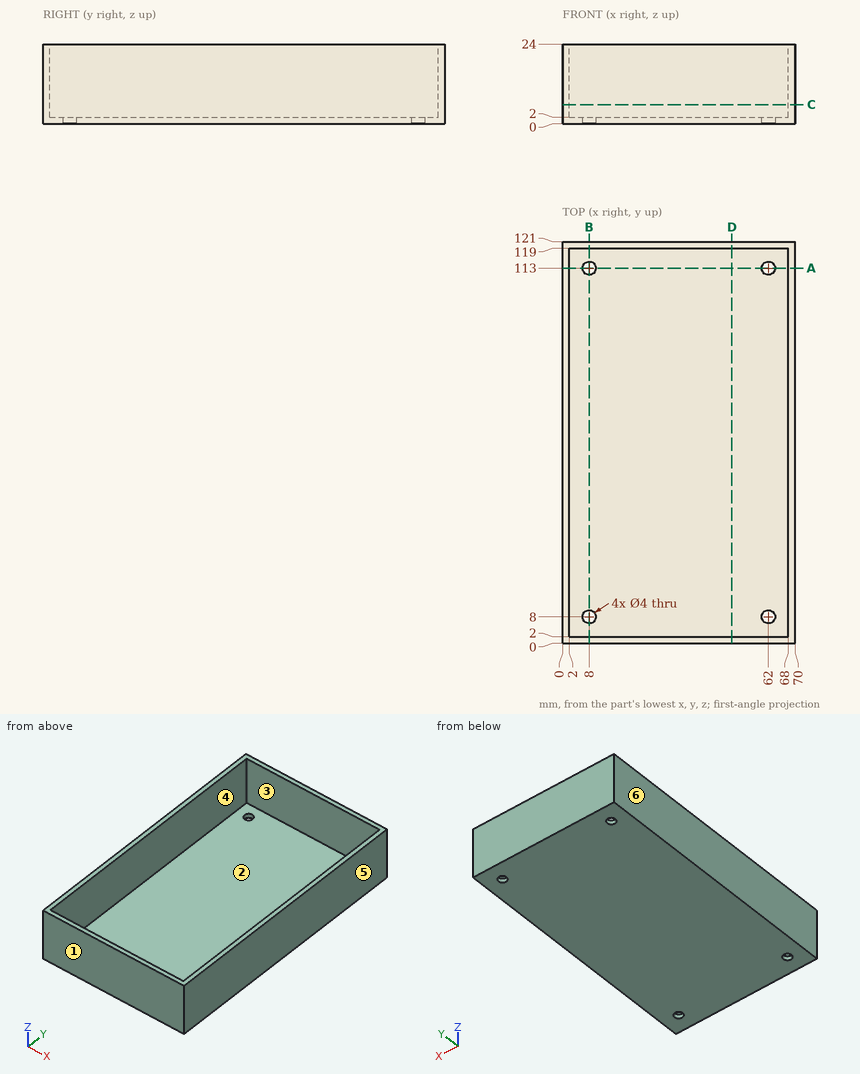
Part print with two shaded views. Sizes in mm from the minimum x, y, z corner. A direction names the side the tool comes from. Give positions to 0.01 mm unless a question says otherwise; leave off trailing zeros. Order: outer loops, then holes, each group sorted by start corner. A loop starts at its lowest first (then second) coordinate and runs counter-clockwise, first axis right, second up.
(1) Flat gauge pins, fed straight in: pin 1 (2.5 mm diameter, centred on x = 8, y = 8, fed in from -Z); pin 2 (8 mm diameter, centred on x = 49, y = 41.5, fed in from +Z). Where does each tip first touch, or does it go through?
(2) Saw through at A-A, the plane y = 113. Give the cut face in (x, z).
(3) Saw through at B-B, the plane x = 8. Give the cut face in (y, z), then the cut area to 3 significant figures.
(4) Drill centre lines: L1, parallel to Y at x = 62, z = 1.5; L2, parallel to Y at x = 7, z = 12; L3, parallel to X at y = 41.5, z = 6. Where is each one in solid material? Low to high.
(5) Saw through at C-C, the plane z = 5.75. Give the cut face in (x, y), then the cut area to 3 significant figures.
(6) Tool access for the marked faces 1 and 2: list every direction of +Z, -Z, +X, -X, +Y, -Y with a clear straight run to the whole face (end or side of a thin tool).
(7) Saw through at D-D, the plane x = 51. Give the cut face in (y, z).
(8) Mould opens along X. For the marked faces 3, 4, 5 and 6 say: released by +X, released by -X, zero draft, split by the parting line, or undercut.
Results found:
1. pin 1: passes through
1. pin 2: stops at z = 2
2. outline: (0, 0) - (6, 0) - (6, 2) - (2, 2) - (2, 24) - (0, 24) - close; (10, 0) - (60, 0) - (60, 2) - (10, 2) - close; (64, 0) - (70, 0) - (70, 24) - (68, 24) - (68, 2) - (64, 2) - close
3. outline: (0, 0) - (6, 0) - (6, 2) - (2, 2) - (2, 24) - (0, 24) - close; (10, 0) - (111, 0) - (111, 2) - (10, 2) - close; (115, 0) - (121, 0) - (121, 24) - (119, 24) - (119, 2) - (115, 2) - close
3. area: 314 mm2
4. L1: y = 0 to 6, 10 to 111, 115 to 121
4. L2: y = 0 to 2, 119 to 121
4. L3: x = 0 to 2, 68 to 70
5. outline: (0, 0) - (70, 0) - (70, 121) - (0, 121) - close; hole (2, 2) - (68, 2) - (68, 119) - (2, 119) - close
5. area: 748 mm2
6. face 1: +Z, -Z, +X, -X, -Y
6. face 2: +Z
7. outline: (0, 0) - (121, 0) - (121, 24) - (119, 24) - (119, 2) - (2, 2) - (2, 24) - (0, 24) - close
8. face 3: undercut
8. face 4: undercut
8. face 5: released by +X
8. face 6: released by -X
